CAD build for the part. Positions are in the model's coordinates, mm. Face numbers are marked on the shaded views. A direction names the side the tool comes from. Give positions to 0.01 mm unless a question says otherwise; leave off trailing zeros. Write each loop counter-clockwise with the first axis right and the second up, starting at its lowest first coordinate (ties: lowest second). Pieces come first, ordered by that corner, then holes. Notation, with made-up numbers: (-34, -30.5) - (-2, -30.5) arc R18 ccw to (-2, -2.5) - close; hole circle Ø2 at (-21.75, -33.75). An arc over 180 degrees is marked (long way). Put each result on its own line as item: value. Start each with the question number.
1. Mould opens along Z. For the marked faces 4, 5, 6 and 7 say: +Z half, -Z half, draft (parallel to the pull), parting line (faces both ways), or undercut.
2. Wall check: line 1 (Z direction, x = 7.25, y = -12.5); line 2 (X direction, y = -13.5, z = -20.75); line 3 (Y direction, x = 2.25, z = 17). Give the ranges that are in metal, low to high.
3. Tool access for the marked faces 1, 2 and 3: list every direction of +Z, -Z, +X, -X, +Y, -Y with a clear straight run to the whole face (end or side of a thin tool).
4. Cut at A-A on z = -9. List the corners of the cut face in (x, y).
5. Drop flat-ended pins along their axis: pin 1 (3 mm diameter, centred on x = 6, z = 20.75, fed in from -Y); pin 2 (5 mm diameter, centred on x = 5, y = 2, fed in from -Z); pin 3 (3 mm diameter, centred on x = 6, z = 22.5, fed in from +Y). Give the stop position or say it passes through.
6. Cut at B-B on x = 6. List the corners of the cut face in (y, z).
7. Cut at C-C on z = 20.75. List the corners of the cut face in (x, y).
8. Cut at D-D on x = 2.5. List the corners of the cut face in (y, z), and give its area (3 significant figures).
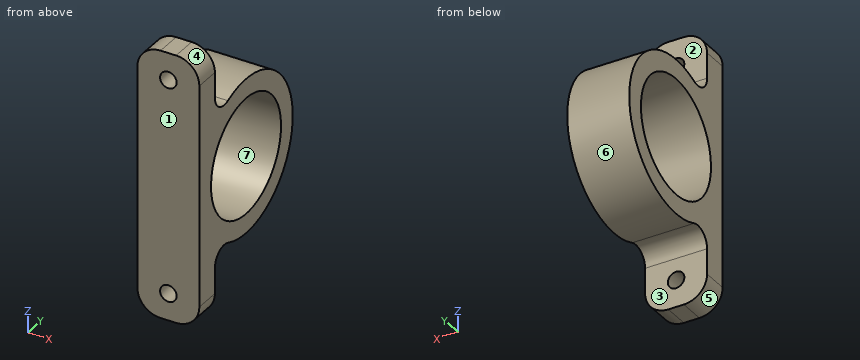
from build123d import *

# Parameters (mm, degrees)
SALIENTE_EXTRUIR1_DEPTH    = 12
CROQUIS2_R                 = 11.25
CORTAR_EXTRUIR1_DEPTH      = 33.32645975
REDONDEO1_R                = 3
REDONDEO2_R                = 4.5
CORTAR_EXTRUIR2_DEPTH      = 10
CORTAR_EXTRUIR2_DEPTH_BACK = 39.013155617
CROQUIS3_R                 = 1.6


with BuildPart() as part:
    # Croquis1 → Saliente-Extruir1 (new body)
    with BuildSketch(Plane(origin=(0, 0, 0), x_dir=(0, 0, -1), z_dir=(1, 0, 0))):
        with BuildLine():
            Line((-26, -15), (26, -15))
            Line((26, -15), (26, -10))
            Line((26, -10), (11.180339887, -10))
            ThreePointArc((11.180339887, -10), (0, 15), (-11.180339887, -10))
            Line((-11.180339887, -10), (-26, -10))
            Line((-26, -10), (-26, -15))
        make_face()
    extrude(amount=SALIENTE_EXTRUIR1_DEPTH)

    # Croquis2 → Cortar-Extruir1 (cut, through all)
    with BuildSketch(Plane.ZY):
        Circle(CROQUIS2_R)
    extrude(amount=-CORTAR_EXTRUIR1_DEPTH, mode=Mode.SUBTRACT)

    # Redondeo1
    redondeo1_edges = [part.edges().sort_by_distance(p)[0] for p in [
        (6, -10, 11.180339887),
        (6, -10, -11.180339887),
    ]]
    fillet(redondeo1_edges, radius=REDONDEO1_R)

    # Redondeo2
    redondeo2_edges = [part.edges().sort_by_distance(p)[0] for p in [
        (12, -12.5, -26),
        (12, -12.5, 26),
        (0, -12.5, -26),
        (0, -12.5, 26),
    ]]
    fillet(redondeo2_edges, radius=REDONDEO2_R)

    # Croquis3 → Cortar-Extruir2 (cut, two sides: drawn at the far end of the back side and taken through both)
    with BuildSketch(Plane(origin=(0, -10, 0), x_dir=(1, 0, 0), z_dir=(0, 1, 0)).offset(-CORTAR_EXTRUIR2_DEPTH_BACK)):
        with Locations(Location((6, 20.75, 0), (0, 0, 90))):
            Circle(CROQUIS3_R)
        with Locations(Location((6, -20.75, 0), (0, 0, 90))):
            Circle(CROQUIS3_R)
    extrude(amount=CORTAR_EXTRUIR2_DEPTH + CORTAR_EXTRUIR2_DEPTH_BACK, mode=Mode.SUBTRACT)


solid = part.part
Report:
1. face 4: +Z half
1. face 5: -Z half
1. face 6: parting line
1. face 7: undercut
2. line 1: z = -26 to -21.75, -19.75 to 19.75, 21.75 to 26
2. line 2: x = 0 to 4.4, 7.6 to 12
2. line 3: y = -15 to -10
3. face 1: +Z, -Z, +X, -X, -Y
3. face 2: +Z, +X, -X, +Y
3. face 3: -Z, +X, -X, +Y
4. outline: (0, -15) - (12, -15) - (12, -6.75) - (0, -6.75) - close; (0, 6.75) - (12, 6.75) - (12, 12) - (0, 12) - close
5. pin 1: passes through
5. pin 2: stops at z = -15
5. pin 3: stops at y = -10
6. outline: (-15, -26) - (-10, -26) - (-10, -22.35) - (-15, -22.35) - close; (-15, -19.15) - (-10, -19.15) - (-10, -16.58) arc R3 cw to (-5.83, -13.82) arc R15 ccw (long way) to (-5.83, 13.82) arc R3 cw to (-10, 16.58) - (-10, 19.15) - (-15, 19.15) - close; (-15, 22.35) - (-10, 22.35) - (-10, 26) - (-15, 26) - close; hole circle Ø22.5 at (0, 0)
7. outline: (0, -15) - (4.4, -15) - (4.4, -10) - (0, -10) - close; (7.6, -15) - (12, -15) - (12, -10) - (7.6, -10) - close
8. outline: (-15, -25.53) - (-10, -25.53) - (-10, -16.58) arc R3 cw to (-5.83, -13.82) arc R15 ccw (long way) to (-5.83, 13.82) arc R3 cw to (-10, 16.58) - (-10, 25.53) - (-15, 25.53) - close; hole circle Ø22.5 at (0, 0)
8. area: 499 mm²
